from build123d import *

# Parameters (mm, degrees)
L_ANGLE_EQUAL_40X40X3_5_DEPTH = 1530
SKETCH16_R                    = 4
CUT_EXTRUDE1_DEPTH            = 1532.045394494


with BuildPart() as part:
    # Sketch13 → L angle (equal) 40X40X3(5) (new body)
    with BuildSketch(Plane(origin=(0, 0, 0), x_dir=(0, 0, -1), z_dir=(1, 0, 0))):
        with BuildLine():
            Line((0, 40), (0, 0))
            Line((0, 0), (40, 0))
            ThreePointArc((40, 0), (39.121320344, 2.121320344), (37, 3))
            Line((37, 3), (9, 3))
            ThreePointArc((9, 3), (4.757359313, 4.757359313), (3, 9))
            Line((3, 9), (3, 37))
            ThreePointArc((3, 37), (2.121320344, 39.121320344), (0, 40))
        make_face()
    extrude(amount=L_ANGLE_EQUAL_40X40X3_5_DEPTH)

    # Sketch16 → Cut-Extrude1 (cut, through all)
    with BuildSketch(Plane.XY):
        with Locations((1500, 20)):
            Circle(SKETCH16_R)
        with Locations((30, 20)):
            Circle(SKETCH16_R)
    extrude(amount=-CUT_EXTRUDE1_DEPTH, mode=Mode.SUBTRACT)


solid = part.part
Check sheet for the modelled part. Datum: model origin and axes. Units: mm. A direction names the side the tool comes from. Coordinates: 2 decimals unless noted, no trailing zeros. Loops run counter-clockwise (first coordinate to the right, second up) from the corner with the lowest first, then second, coordinate; pieces in that order, holes last. Notation, with made-up numbers: (37, 13) -> (73, 13) arc R5 cw to (73, 18) -> close; hole circle Ø10 at (13.25, 24). An arc over 180 degrees is marked (long way). Answer in a Markdown table with one row per item.
1. Access from +Z, -Z, +X, -X, +Y, -Y to the whole of each face (thin tool, end or side, straight path). Record for faces 1 (the face through (1530, 10, -2)), 2 (the face through (754, 3, -23)).
Check values:
| item | result |
|---|---|
| face 1 | +Z, -Z, +X, +Y, -Y |
| face 2 | -Z, +X, -X, +Y |
2. Sectioned sample at C-C, the plane y = 30. Record the boundary of the cut face in (x, z).
Check values:
| item | result |
|---|---|
| outline | (0, -3) -> (1530, -3) -> (1530, 0) -> (0, 0) -> close |
3. Go/stop test with flat-tipped pins: pin 1 (22.5 mm diameter, centred on x = 1107, z = -17.5, fed in from +Y); pin 2 (12 mm diameter, centred on y = 5, z = -11, fed in from +X); pin 3 (1 mm diameter, centred on x = 219.5, z = -30.5, fed in from +Y); pin 4 (10.5 mm diameter, centred on x = 1500, y = 20, fed in from -Z). Record where each tip stops, or that it passes through.
Check values:
| item | result |
|---|---|
| pin 1 | stops at y = 3.67 |
| pin 2 | stops at x = 1530 |
| pin 3 | stops at y = 3 |
| pin 4 | stops at z = -3 |
4. Sectioned sample at A-A, the plane x = 1287.5. Record the boundary of the cut face in (y, z), then the cut area to 3 significant figures.
Check values:
| item | result |
|---|---|
| outline | (0, -40) arc R3 ccw to (3, -37) -> (3, -9) arc R6 cw to (9, -3) -> (37, -3) arc R3 ccw to (40, 0) -> (0, 0) -> close |
| area | 235 mm2 |
5. Sectioned sample at B-B, the plane z = -19. Record the boundary of the cut face in (x, y), then the cut area to 3 significant figures.
Check values:
| item | result |
|---|---|
| outline | (0, 0) -> (1530, 0) -> (1530, 3) -> (0, 3) -> close |
| area | 4,590 mm2 |
6. Material ranges on line 1 along Y through (x, z) = (1500, -1.3); line 2 along Y through (x, z) = (621, -36); line 3 along Y through (x, z) = (1500, -0.65), recorded low to high. Write a range as [from, to].
Check values:
| item | result |
|---|---|
| line 1 | y = [0, 16], [24, 39.7] |
| line 2 | y = [0, 3] |
| line 3 | y = [0, 16], [24, 39.93] |
